Check sheet for the modelled part. Datum: model origin and axes. Units: mm. Face numbers are marked on the shaded views. Coordinates: 2 decimals unless noted, no trailing zeros. Order: outer loops, then holes, each group sorted by start corner. A loop starts at its lowest first (then second) coordinate and runs counter-clockwise, first axis right, second up.
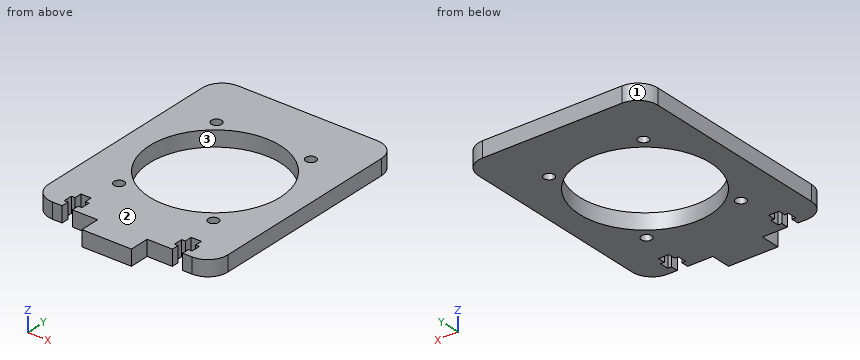
from build123d import *

# Parameters (mm, degrees)
SKETCH1_W           = 115
SKETCH1_H           = 150
SKETCH1_R           = 42
SKETCH1_R_2         = 3.3
BOSS_EXTRUDE1_DEPTH = 10
CUT_EXTRUDE1_DEPTH  = 96.032889044
BOSS_EXTRUDE2_DEPTH = 12.7
FILLET1_R           = 12.8


with BuildPart() as part:
    # Sketch1 → Boss-Extrude1 (new body)
    with BuildSketch(Plane.XY):
        Rectangle(SKETCH1_W, SKETCH1_H)
        Circle(SKETCH1_R, mode=Mode.SUBTRACT)
        with Locations((-30.226879089, 39.426364029)):
            Circle(SKETCH1_R_2, mode=Mode.SUBTRACT)
        with Locations((30.226879089, 39.426364029)):
            Circle(SKETCH1_R_2, mode=Mode.SUBTRACT)
        with Locations((30.226879089, -39.426364029)):
            Circle(SKETCH1_R_2, mode=Mode.SUBTRACT)
        with Locations((-30.226879089, -39.426364029)):
            Circle(SKETCH1_R_2, mode=Mode.SUBTRACT)
    extrude(amount=BOSS_EXTRUDE1_DEPTH)

    # Sketch2 → Cut-Extrude1 (cut, through all)
    with BuildSketch(Plane(origin=(0, 0, 0), x_dir=(-1, 0, 0), z_dir=(0, 0, -1))):
        Polygon((-38.65, -75), (-32.05, -75), (-32.05, -70.3), (-29.686, -70.3), (-29.686, -64.46), (-32.05, -64.46), (-32.05, -59.76), (-38.65, -59.76), (-38.65, -64.46), (-41.014, -64.46), (-41.014, -70.3), (-38.65, -70.3), align=None)
        Polygon((32.05, -75), (32.05, -70.3), (29.686, -70.3), (29.686, -64.46), (32.05, -64.46), (32.05, -59.76), (38.65, -59.76), (38.65, -64.46), (41.014, -64.46), (41.014, -70.3), (38.65, -70.3), (38.65, -75), align=None)
    extrude(amount=-CUT_EXTRUDE1_DEPTH, mode=Mode.SUBTRACT)

    # Sketch4 → Boss-Extrude2 (add)
    with BuildSketch(Plane.XZ.offset(75)):
        Polygon((0, 0), (15.875, 0), (15.875, 10), (-15.875, 10), (-15.875, 0), align=None)
    extrude(amount=BOSS_EXTRUDE2_DEPTH)

    # Fillet1
    fillet1_edges = [part.edges().sort_by_distance(p)[0] for p in [
        (57.5, -75, 5),
        (-57.5, -75, 5),
        (-57.5, 75, 5),
        (57.5, 75, 5),
    ]]
    fillet(fillet1_edges, radius=FILLET1_R)


solid = part.part
(1) Go/stop test with flat-tipped pins: P1, Ø5, axis at y = -73, z = 2.5, coming from the -X side; P2, Ø3, axis at y = -68.5, z = 7, coming from the +X side; P3, Ø3, axis at y = -79, z = 7, coming from the -X side (3 decimals). Record where each tip stops, or that it passes through.
Filled in:
P1: stops at x = -54.44
P2: stops at x = 56.57
P3: stops at x = -15.875
(2) Thickness scan on probe 1 along X at (y, z) = (-62.5, 6); probe 2 along X at (y, z) = (-37.5, 7); probe 3 along Y at (x, z) = (-32, 0.75). Record the ranges inside material, lowest first.
Filled in:
probe 1: x = -57.5 to -38.65, -32.05 to 32.05, 38.65 to 57.5
probe 2: x = -57.5 to -32.91, -27.55 to -18.91, 18.91 to 27.55, 32.91 to 57.5
probe 3: y = -75 to -70.3, -64.46 to -42.21, -36.64 to -27.2, 27.2 to 36.64, 42.21 to 75
(3) Cross-section at D-D (x = -48). Enter the section's corners in (y, z).
Filled in:
outline: (-74.57, 0) - (74.57, 0) - (74.57, 10) - (-74.57, 10) - close
(4) Cross-section at A-A (y = 0). Enter the section's corners in (x, z).
Filled in:
outline: (-57.5, 0) - (-42, 0) - (-42, 10) - (-57.5, 10) - close; (42, 0) - (57.5, 0) - (57.5, 10) - (42, 10) - close
(5) Cross-section at C-C (z = 1.5). Count the separate pieces of the cut face and the enclosed holes in it, and give its area (3 significant figures).
Filled in:
separate pieces: 1
enclosed holes: 5
area: 11,600 mm2
(6) Release check for a two-part mould opening along Y. For the marked faces 1, 2 and 3 record: +Y half, -Y half, draft (parallel to the pull), parting line (faces both ways), or undercut.
Filled in:
face 1: +Y half
face 2: draft
face 3: undercut
(7) Cross-section at B-B (x = 0). Enter the section's corners in (y, z), and give its area (3 significant figures).
Filled in:
outline: (-87.7, 0) - (-42, 0) - (-42, 10) - (-87.7, 10) - close; (42, 0) - (75, 0) - (75, 10) - (42, 10) - close
area: 787 mm2
